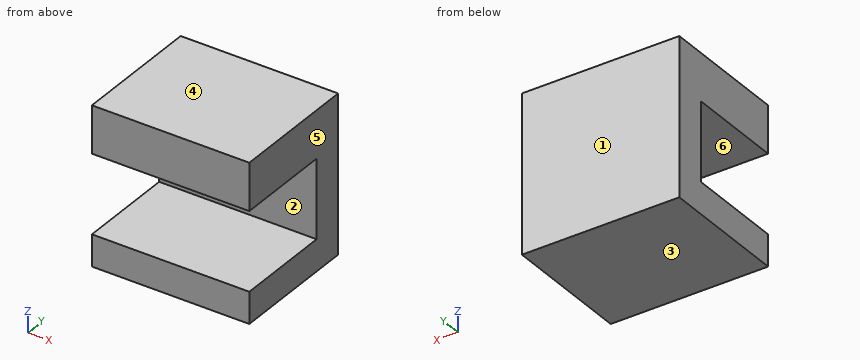
```python
from build123d import *

# Parameters (mm, degrees)
BOSS_EXTRUDE1_DEPTH = 12.5
BOSS_EXTRUDE4_DEPTH = 20


with BuildPart() as part:
    # Sketch1 → Boss-Extrude1 (new body)
    with BuildSketch(Plane(origin=(0, 0, 0), x_dir=(1, 0, 0), z_dir=(0, 1, 0))):
        Polygon((-2.564516129, 3.29516129), (14.435483871, 3.29516129), (14.435483871, -2.70483871), (-5.564516129, -2.70483871), (-5.564516129, 3.29516129), (-4.064516129, 3.29516129), align=None)
    extrude(amount=BOSS_EXTRUDE1_DEPTH)

    # Sketch2 → Boss-Extrude4 (add)
    with BuildSketch(Plane(origin=(14.435483871, 0, 0), x_dir=(0, 0, -1), z_dir=(1, 0, 0))):
        Polygon((-2.70483871, 12.5), (13.29516129, 12.5), (13.29516129, 0), (17.29516129, 0), (17.29516129, 12.5), (17.29516129, 16.5), (-2.70483871, 16.5), align=None)
    extrude(amount=-BOSS_EXTRUDE4_DEPTH)


solid = part.part
```
Can you work these out from the model? Positions are in its coordinate system, mm. Face numbers are marked on the shaded views. A direction names the side the tool comes from. Round coordinates to 2 decimals unless told otherwise and drop trailing zeros. Loops run counter-clockwise (first coordinate to the right, second up) from the corner with the lowest first, then second, coordinate; pieces in that order, holes last. Notation, with made-up numbers: (-8.75, 3.5) -> (46.25, 3.5) arc R17 ccw to (46.25, 13.5) -> close; hole circle Ø11 at (28, -17). An arc over 180 degrees is marked (long way). One line per item, written item: value. Start each with the question number.
1. For the marked faces 5 and 6, which set-ups out of +Z, -Z, +X, -X, +Y, -Y let a thin tool reach every point of the face, with its end or its side?
2. If we mould it in two halves opening along Z, with no side actions, what happens to the marked faces 1, 2, 3 and 4? For each: pulls with the +Z half, pulls with the -Z half, needs draft (parallel to the pull), parting line crosses it, or undercut.
3. For pin 1 (2 mm diameter, centred on x = 12.5, z = -6, fed in from -Y); pin 2 (5 mm diameter, centred on y = 3, z = -12.5, fed in from -X), each with a flat end and sliding along its axis, tell me the tip position at first contact or that it passes through.
4. If we section it at B-B, the plane x = 7: Write out the boundary of the cut face in (y, z), then the cut area to 3 significant figures.
5. If we section it at A-A, the plane y = 9: Write out the boundary of the cut face in (x, z).
6. If we section it at C-C, the plane z = -4.5: Write out the boundary of the cut face in (x, y), then the cut area to 3 significant figures.
7. If I drill on probe 1 along Z at (x, y) = (12, 7.75); probe 2 along Y at (x, z) = (7, -10.75), over which ranges is the centre line in solid material (lowest first)?
Calculated:
1. face 5: +Z, -Z, +X, +Y, -Y
1. face 6: +X, -X, -Y
2. face 1: needs draft
2. face 2: undercut
2. face 3: pulls with the -Z half
2. face 4: pulls with the +Z half
3. pin 1: stops at y = 12.5
3. pin 2: stops at x = -5.56
4. outline: (0, -17.3) -> (16.5, -17.3) -> (16.5, 2.7) -> (0, 2.7) -> (0, -3.3) -> (12.5, -3.3) -> (12.5, -13.3) -> (0, -13.3) -> close
4. area: 205 mm²
5. outline: (-5.56, -17.3) -> (14.44, -17.3) -> (14.44, -13.3) -> (-5.56, -13.3) -> close; (-5.56, -3.3) -> (14.44, -3.3) -> (14.44, 2.7) -> (-5.56, 2.7) -> close
6. outline: (-5.56, 12.5) -> (14.44, 12.5) -> (14.44, 16.5) -> (-5.56, 16.5) -> close
6. area: 80.0 mm²
7. probe 1: z = -17.3 to -13.3, -3.3 to 2.7
7. probe 2: y = 12.5 to 16.5
